Read the model definition and answer for the solid it produces. Units are mm, in the model's axes. Face numbers are marked on the shaded views. Give positions to 0.01 mm unless a question says otherwise; leave off trailing zeros. Order: outer loops, then holes, each group sorted by start corner. A loop starts at its lowest first (then second) coordinate and runs counter-clockwise, first axis right, second up.
```python
from build123d import *

# Parameters (mm, degrees)
SKETCH1_R           = 5
BOSS_EXTRUDE1_DEPTH = 26
CUT_EXTRUDE1_DEPTH  = 3
FILLET1_R           = 1


with BuildPart() as part:
    # Sketch1 → Boss-Extrude1 (new body)
    with BuildSketch(Plane(origin=(0, 0, 0), x_dir=(1, 0, 0), z_dir=(0, 1, 0))):
        with Locations(Location((0, 0, 0), (0, 0, 90))):
            Circle(SKETCH1_R)
    extrude(amount=BOSS_EXTRUDE1_DEPTH)

    # Sketch2 → Cut-Revolve1 (revolve, cut)
    with BuildSketch(Plane.XY):
        with BuildLine():
            Line((0, -4.1), (0, 4.1))
            ThreePointArc((0, 4.1), (4.1, 0), (0, -4.1))
        make_face()
    revolve(axis=Axis((0, -4.1, 0), (0, 1, 0)), mode=Mode.SUBTRACT)

    # Sketch4 → Revolve1 (revolve)
    with BuildSketch(Plane(origin=(0, 2, 0), x_dir=(1, 0, 0), z_dir=(0, 1, 0))):
        with BuildLine():
            Line((0, 6), (0, 5))
            ThreePointArc((0, 5), (0.5, 4.974937186), (0.994987437, 4.9))
            ThreePointArc((0.994987437, 4.9), (0.741619849, 5.670820393), (0, 6))
        make_face()
    revolve1 = revolve(axis=Axis((0, 2, 0), (0, 0, -1)))

    # Sketch5 → Cut-Extrude1 (cut)
    with BuildSketch(Plane(origin=(0, 26, 0), x_dir=(1, 0, 0), z_dir=(0, 1, 0))):
        Polygon((-4.041451884, 0), (-2.020725942, -3.5), (2.020725942, -3.5), (4.041451884, 0), (2.020725942, 3.5), (-2.020725942, 3.5), align=None)
    extrude(amount=-CUT_EXTRUDE1_DEPTH, mode=Mode.SUBTRACT)

    # Mirror1: Revolve1 across plane
    add(revolve1.mirror(Plane.XY))

    # Fillet1
    # the kernel refuses this fillet: 1 mm, written as the material it takes off along each edge
    with BuildSketch(Plane(origin=(0, 0, 0), x_dir=(0, 0, -1), z_dir=(1, 0, 0))) as fillet1_piece_1:
        with BuildLine():
            CenterArc((4, 0.994987437), FILLET1_R, 275.739170477, 84.260829523)
            Line((4.1, 0), (4.102, -0.019899749))
            ThreePointArc((4.102, -0.019899749), (4.55, -0.02), (5, -0.02))
            Line((5, -0.02), (5.02, 0))
            Line((5.02, 0), (5.02, 0.994987437))
            Line((5.02, 0.994987437), (5, 0.994987437))
        make_face()
    revolve(axis=Axis((0, 0, 0), (0, 1, 0)), mode=Mode.SUBTRACT)


solid = part.part
```
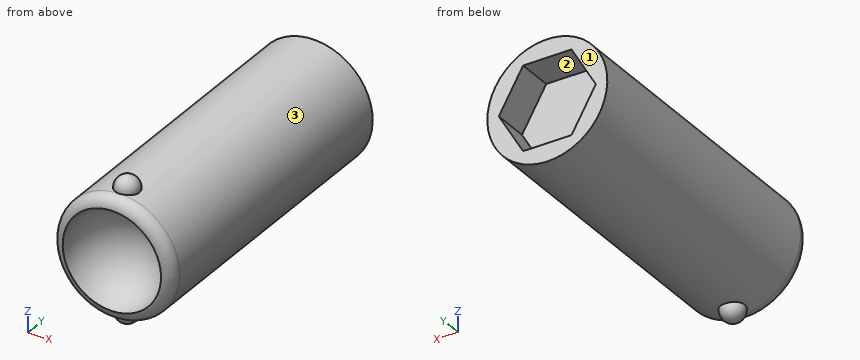
1) The part is cut by section A-A on y = 23.5. Determine the outline of the cut face in (x, z).
Final values:
outline: circle Ø10 at (0, 0); hole (-4.04, 0) - (-2.02, -3.5) - (2.02, -3.5) - (4.04, 0) - (2.02, 3.5) - (-2.02, 3.5) - close
2) For a pull along X with two mould halves and no side action, classify the marked faces 1, 2 and 3 as released by +X, released by -X, zero draft, split by the parting line, or undercut.
Final values:
face 1: zero draft
face 2: undercut
face 3: split by the parting line
3) Given pin 1 (1.5 mm diameter, centred on x = 2, z = 1.5, fed in from -Y); pin 2 (0.9 mm diameter, centred on x = 0.5, y = 24, fed in from -Z); pin 3 (0.9 mm diameter, centred on x = 0, y = 25, fed in from +Z), each flat-ended and moving along its own axis, determine where each tip first touches the part or whether it passes through.
Final values:
pin 1: stops at y = 2.5
pin 2: stops at z = -5
pin 3: stops at z = 5
4) Consider L1, parallel to X at y = 23.5, z = -1.5; L2, parallel to X at y = 23.5, z = 2; L3, parallel to Z at x = -1, y = 21. Determine where each line is inside the solid, lowest interval first.
Final values:
L1: x = -4.77 to -3.18, 3.18 to 4.77
L2: x = -4.58 to -2.89, 2.89 to 4.58
L3: z = -4.9 to 4.9
